Build history of the part. All positions in model axes, mm. A direction names the side the tool comes from. Give positions to 0.01 mm unless a question says otherwise; leave off trailing zeros. Loops run counter-clockwise (first coordinate to the right, second up) from the corner with the lowest first, then second, coordinate; pieces in that order, holes last.
1) Band-saw the part on A-A on x = -11.15. List the corners of the cut face in (y, z).
2) Flat gauge pins, fed straight in: P1, Ø0.6, axis at x = 10.5, z = 1, coming from the -Y side; P2, Ø2.5, axis at y = -5, z = 1.5, coming from the -X side; P3, Ø4, axis at y = 0.85, z = -9.88, coming from the -X side; P4, Ø3.5, axis at y = -6.5, z = 2, coming from the +X side. Where does each tip first touch, or does it go through?
3) Band-saw the part on D-D on z = 0.75. List the corners of the cut face in (x, y) (3 decimals).
4) Wall check: line 1 (X direction, y = 0, z = -1.25); line 2 (Y direction, x = -11.15, z = 1.2); line 3 (Z direction, x = -11, y = -10.5). Give the ranges that are in metal, low to high.
5) Two-plate mould, pull along Y, no slides. Class faces 6 (the cylindrical face through (-13.965, 1.944, -0.301)), 7 (the cylindrical face through (-15.01, -0.011, -7.797)), 8 (the cylindrical face through (-0.22, 7.467, -14.208)): +Y half, -Y half, draft (parallel to the pull), parting line (faces both ways), or undercut.
6) 3-axis set-ups, long thin cutter, end or side, ignore diameter. For faces 1 (the flat face through (12.75, 0, 1)), 2 (the cylindrical face through (9.035, -2.371, 1.479)), 3 (the cylindrical face through (0.2, 4.31, -0.57)), 4 (the cylindrical face through (-12.865, -14.571, 1.479)), 5 (the flat face through (-11, -14.872, 1)): which of +Z, -Z, +X, -X, +Y, -Y reach the whole face in a straight line?
7) Band-saw the part on B-B on z = -10. State how many separate pieces and enclosed holes the cut face has, then the cut area to 3 significant figures.
8) Band-saw the part on C-C on x = 3. List the corners of the cut face in (y, z).
```python
from build123d import *

# Parameters (mm, degrees)
SKETCH1_R            = 1.125
BOSS_EXTRUDE1_DEPTH  = 3
BOSS_EXTRUDE2_DEPTH  = 3
SKETCH4_R            = 2.25
BOSS_EXTRUDE4_DEPTH  = 1.5
BOSS_EXTRUDE5_START  = 28.5
BOSS_EXTRUDE5_DEPTH  = 28.5
SKETCH8_W            = 28.5
SKETCH8_H            = 3
BOSS_EXTRUDE13_DEPTH = 2.443258406
FILLET1_R            = 2
FILLET2_R            = 1


with BuildPart() as part:
    # Sketch1 → Boss-Extrude1 (new body)
    with BuildSketch(Plane.XY):
        with BuildLine():
            Line((-13.15, 3.327838927), (-13.15, -13.87167957))
            ThreePointArc((-13.15, -13.87167957), (-12.857106781, -14.578786352), (-12.15, -14.87167957))
            Line((-12.15, -14.87167957), (-10.15, -14.87167957))
            ThreePointArc((-10.15, -14.87167957), (-9.442893219, -14.578786352), (-9.15, -13.87167957))
            Line((-9.15, -13.87167957), (-9.15, -2.961805456))
            ThreePointArc((-9.15, -2.961805456), (-7.978427125, -0.133378332), (-5.15, 1.038194544))
            Line((-5.15, 1.038194544), (6.75, 1.038194544))
            ThreePointArc((6.75, 1.038194544), (8.164213562, 0.452408106), (8.75, -0.961805456))
            Line((8.75, -0.961805456), (8.75, -1.67167957))
            ThreePointArc((8.75, -1.67167957), (9.042893219, -2.378786352), (9.75, -2.67167957))
            Line((9.75, -2.67167957), (11.75, -2.67167957))
            ThreePointArc((11.75, -2.67167957), (12.457106781, -2.378786352), (12.75, -1.67167957))
            Line((12.75, -1.67167957), (12.75, 3.327838927))
            Line((12.75, 3.327838927), (-13.15, 3.327838927))
        make_face()
        with Locations((-11.15, -12.87167957)):
            Circle(SKETCH1_R, mode=Mode.SUBTRACT)
        with Locations((10.75, -0.67167957)):
            Circle(SKETCH1_R, mode=Mode.SUBTRACT)
    extrude(amount=BOSS_EXTRUDE1_DEPTH)


with BuildPart() as body_2:
    # Sketch2 → Boss-Extrude2 (new body)
    with BuildSketch(Plane(origin=(12.75, 0, 0), x_dir=(0, 0, -1), z_dir=(1, 0, 0))):
        with BuildLine():
            Line((0, -0.048364378), (0, 3.327838927))
            Line((0, 3.327838927), (-3, 3.327838927))
            Line((-3, 3.327838927), (-3, 1.403074886))
            ThreePointArc((-3, 1.403074886), (-1.469520823, 0.740353088), (0, -0.048364378))
        make_face()
    boss_extrude2 = extrude(amount=BOSS_EXTRUDE2_DEPTH)


with BuildPart() as body_3:
    # Sketch4 → Boss-Extrude4 (new body)
    with BuildSketch(Plane.ZY.offset(-15.75)):
        with BuildLine():
            Line((-14.619360276, 0.851097333), (-14.619360276, 6.251097333))
            ThreePointArc((-14.619360276, 6.251097333), (-14.218539822, 7.452190493), (-13.176735496, 8.171860948))
            ThreePointArc((-13.176735496, 8.171860948), (-12.655081911, 8.532697951), (-12.455426242, 9.134747301))
            ThreePointArc((-12.455426242, 9.134747301), (-12.072768819, 8.089517784), (-11.108469635, 7.533593094))
            Line((-11.108469635, 7.533593094), (-1.19901898, 5.78628958))
            ThreePointArc((-1.19901898, 5.78628958), (-1.112526545, 5.774902634), (-1.025370803, 5.771097333))
            Line((-1.025370803, 5.771097333), (2.544576896, 5.771097333))
            Line((2.544576896, 5.771097333), (3, 5.763220708))
            Line((3, 5.763220708), (3, 1.403074886))
            ThreePointArc((3, 1.403074886), (-2.995287542, -2.222261242), (-7.359906948, -7.702829842))
            Line((-7.359906948, -7.702829842), (-13.016847846, -2.703672769))
            ThreePointArc((-13.016847846, -2.703672769), (-14.200215671, -1.098546004), (-14.619360276, 0.851097333))
        make_face()
        with Locations((-9.875423105, 0.851097333)):
            Circle(SKETCH4_R, mode=Mode.SUBTRACT)
    boss_extrude4 = extrude(amount=BOSS_EXTRUDE4_DEPTH)

    # Sketch5 → Boss-Extrude5 (add)
    with BuildSketch(Plane.ZY.offset(-14.25).offset(BOSS_EXTRUDE5_START)):
        with BuildLine():
            Line((0, 4.911114143), (0, 5.771097333))
            Line((0, 5.771097333), (-1.025370803, 5.771097333))
            ThreePointArc((-1.025370803, 5.771097333), (-1.112526545, 5.774902634), (-1.19901898, 5.78628958))
            Line((-1.19901898, 5.78628958), (-11.108470351, 7.533589032))
            ThreePointArc((-11.108470351, 7.533589032), (-12.072769301, 8.089518357), (-12.455426242, 9.134747301))
            ThreePointArc((-12.455426242, 9.134747301), (-12.655081911, 8.532697951), (-13.176735496, 8.171860948))
            ThreePointArc((-13.176735496, 8.171860948), (-14.218539822, 7.452190493), (-14.619360276, 6.251097333))
            Line((-14.619360276, 6.251097333), (-14.619360276, 5.411114143))
            ThreePointArc((-14.619360276, 5.411114143), (-14.472913667, 5.057560752), (-14.119360276, 4.911114143))
            Line((-14.119360276, 4.911114143), (0, 4.911114143))
        make_face()
    extrude(amount=-BOSS_EXTRUDE5_DEPTH)


with BuildPart() as part_1:
    add(part.part)

    # Mirror4: Boss-Extrude2, Boss-Extrude4 across plane
    add(boss_extrude2.mirror(Plane(origin=(0, 0, 0), x_dir=(0, 0, 1), z_dir=(1, 0, 0))))
    add(boss_extrude4.mirror(Plane(origin=(0, 0, 0), x_dir=(0, 0, 1), z_dir=(1, 0, 0))))

    add(body_2.part)  # Boss-Extrude13 merges body 2

    add(body_3.part)  # Boss-Extrude13 merges body 3
    # Sketch8 → Boss-Extrude13 (add)
    with BuildSketch(Plane(origin=(0, 3.327838927, 0), x_dir=(1, 0, 0), z_dir=(0, 1, 0))):
        with Locations((0, -1.5)):
            Rectangle(SKETCH8_W, SKETCH8_H)
    extrude(amount=BOSS_EXTRUDE13_DEPTH)

    # Fillet1
    fillet1_edges = [part_1.edges().sort_by_distance(p)[0] for p in [
        (0, 4.911114143, 0),
    ]]
    fillet(fillet1_edges, radius=FILLET1_R)

    # Fillet2
    # the kernel refuses this fillet: 1 mm, written as the material it adds along each edge
    with BuildSketch(Plane(origin=(14.25, -2.548364378, 0), x_dir=(0, 0, -1), z_dir=(0, 1, 0))) as fillet2_piece_1_section:
        with BuildLine():
            CenterArc((FILLET2_R, FILLET2_R), FILLET2_R, 180, 90)
            Line((0, FILLET2_R), (0, 0))
            Line((0, 0), (FILLET2_R, 0))
        make_face()
    fillet2_piece_1 = extrude(amount=7.959478521, mode=Mode.PRIVATE)
    fillet2_piece_1 = fillet2_piece_1 - Plane(origin=(13.964239779, -17.148902667, 10.124576895), x_dir=(0, 0.9335275549954881, -0.35850565415924185), z_dir=(1, 0, 0)) * Cylinder(19.872983346, 20, mode=Mode.PRIVATE)
    add(fillet2_piece_1)
    with BuildSketch(Plane(origin=(-14.25, -2.548364378, 0), x_dir=(1, 0, 0), z_dir=(0, 1, 0))) as fillet2_piece_2_section:
        with BuildLine():
            CenterArc((FILLET2_R, FILLET2_R), FILLET2_R, 180, 90)
            Line((0, FILLET2_R), (0, 0))
            Line((0, 0), (FILLET2_R, 0))
        make_face()
    fillet2_piece_2 = extrude(amount=7.959478521, mode=Mode.PRIVATE)
    fillet2_piece_2 = fillet2_piece_2 - Plane(origin=(-13.964240251, -17.148902667, 10.124576895), x_dir=(0, 0.9335275549956203, -0.3585056541588977), z_dir=(1, 0, 0)) * Cylinder(19.872983346, 20, mode=Mode.PRIVATE)
    add(fillet2_piece_2)


solid = part_1.part
```
Findings below:
1. outline: (-14.87, 0) - (-14, 0) - (-14, 3) - (-14.87, 3) - close; (-11.75, 0) - (2.91, 0) arc R2 cw to (4.91, -2) - (4.91, -14.12) arc R0.5 ccw to (5.41, -14.62) - (6.25, -14.62) arc R2 ccw to (8.17, -13.18) arc R1 cw to (9.13, -12.46) arc R1.63 cw to (7.53, -11.11) - (5.79, -1.2) arc R1 cw to (5.77, -1.03) - (5.77, 3) - (-11.75, 3) - close
2. P1: stops at y = -2.67
2. P2: stops at x = -13.15
2. P3: passes through
2. P4: stops at x = -9.15
3. outline: (-15.75, 0.374) - (-13.15, 0.374) - (-13.15, -13.872) arc R1 ccw to (-12.15, -14.872) - (-10.15, -14.872) arc R1 ccw to (-9.15, -13.872) - (-9.15, -2.962) arc R4 cw to (-5.15, 1.038) - (6.75, 1.038) arc R2 cw to (8.75, -0.962) - (8.75, -1.672) arc R1 ccw to (9.75, -2.672) - (11.75, -2.672) arc R1 ccw to (12.75, -1.672) - (12.75, 0.374) - (15.75, 0.374) - (15.75, 5.771) - (-15.75, 5.771) - close; hole circle Ø2.25 at (-11.15, -12.872); hole circle Ø2.25 at (10.75, -0.672)
4. line 1: x = -15.75 to -14.25, 14.25 to 15.75
4. line 2: y = -14.87 to -14, -11.75 to 5.77
4. line 3: z = 0 to 3
5. face 6: draft
5. face 7: undercut
5. face 8: +Y half
6. face 1: +Z, +X, -Y
6. face 2: +Z, -Z, -Y
6. face 3: -Z, -Y
6. face 4: +Z, -Z, -X, -Y
6. face 5: +Z, -Z, +X, -X, -Y
7. separate pieces: 3
7. enclosed holes: 0
7. area: 93.8 mm2
8. outline: (1.04, 0) - (2.91, 0) arc R2 cw to (4.91, -2) - (4.91, -14.12) arc R0.5 ccw to (5.41, -14.62) - (6.25, -14.62) arc R2 ccw to (8.17, -13.18) arc R1 cw to (9.13, -12.46) arc R1.63 cw to (7.53, -11.11) - (5.79, -1.2) arc R1 cw to (5.77, -1.03) - (5.77, 3) - (1.04, 3) - close
